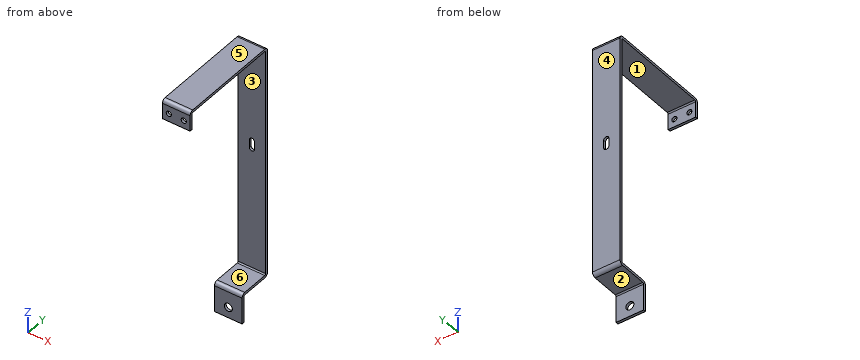
```python
from build123d import *

# Parameters (mm, degrees)
SKETCH1_W                    = 17.5
SKETCH1_H                    = 10
BASE_FLANGE1_DEPTH           = 1.6
EDGE_FLANGE1_DEPTH           = 17.5
EDGE_FLANGE2_STRIP_W         = 7.8732
EDGE_FLANGE2_STRIP_H         = 1.6
EDGE_FLANGE2_STRIP_CUT_DEPTH = 17.5
EDGE_FLANGE2_DEPTH           = 17.5
EDGE_FLANGE3_STRIP_W         = 7.8732
EDGE_FLANGE3_STRIP_H         = 1.6
EDGE_FLANGE3_STRIP_CUT_DEPTH = 17.5
EDGE_FLANGE3_DEPTH           = 17.5
F_4_CLEARANCE_HOLE1_D        = 3.2639
F_4_CLEARANCE_HOLE1_DEPTH    = 1.6
F_4_CLEARANCE_HOLE1_TIP      = 0.980574487
CUT_EXTRUDE3_DEPTH           = 1.6
EDGE_FLANGE4_STRIP_W         = 7.8732
EDGE_FLANGE4_STRIP_H         = 1.6
EDGE_FLANGE4_STRIP_CUT_DEPTH = 17.5
EDGE_FLANGE4_DEPTH           = 17.5
F_10_CLEARANCE_HOLE1_D       = 5.1054
F_10_CLEARANCE_HOLE1_DEPTH   = 7.6
F_10_CLEARANCE_HOLE1_TIP     = 1.533816902


# Sheet-metal steps are written as plain solids
with BuildPart() as part:
    # Sketch1 → Base-Flange1 (new body)
    with BuildSketch(Plane(origin=(0, 0, 0), x_dir=(1, 0, 0), z_dir=(0, 1, 0))):
        Rectangle(SKETCH1_W, SKETCH1_H)
    extrude(amount=BASE_FLANGE1_DEPTH)

    # Edge-Flange1 section (across the edge) → Edge-Flange1 (add)
    with BuildSketch(Plane(origin=(-8.75, 1.6, 5.7366), x_dir=(0, 0, -1), z_dir=(1, 0, 0))):
        with BuildLine():
            Line((-1.6, 0.7366), (-1.6, 65.4))
            Line((-1.6, 65.4), (0, 65.4))
            Line((0, 65.4), (0, 0.7366))
            ThreePointArc((0, 0.7366), (0.215745145, 0.215745145), (0.7366, 0))
            Line((0.7366, 0), (0.7366, -1.6))
            ThreePointArc((0.7366, -1.6), (-0.915625705, -0.915625705), (-1.6, 0.7366))
        make_face()
    extrude(amount=EDGE_FLANGE1_DEPTH)

    # Edge-Flange2 strip (across the edge) → Edge-Flange2 strip cut (cut)
    with BuildSketch(Plane(origin=(-8.75, 67, 5.7366), x_dir=(0, -1, 0), z_dir=(1, 0, 0))):
        with Locations((-1.6, -0.8)):
            Rectangle(EDGE_FLANGE2_STRIP_W, EDGE_FLANGE2_STRIP_H)
    extrude(amount=EDGE_FLANGE2_STRIP_CUT_DEPTH, mode=Mode.SUBTRACT)

    # Edge-Flange2 section (across the edge) → Edge-Flange2 (add)
    with BuildSketch(Plane(origin=(-8.75, 67, 5.7366), x_dir=(0, -1, 0), z_dir=(1, 0, 0))):
        with BuildLine():
            Line((0, 0.7366), (0, 147.4))
            Line((0, 147.4), (1.6, 147.4))
            Line((1.6, 147.4), (1.6, 0.7366))
            ThreePointArc((1.6, 0.7366), (1.815745145, 0.215745145), (2.3366, 0))
            Line((2.3366, 0), (2.3366, -1.6))
            ThreePointArc((2.3366, -1.6), (0.684374295, -0.915625705), (0, 0.7366))
        make_face()
    extrude(amount=EDGE_FLANGE2_DEPTH)

    # Edge-Flange3 strip (across the edge) → Edge-Flange3 strip cut (cut)
    with BuildSketch(Plane(origin=(-8.75, 65.4, -141.6634), x_dir=(0, 0, 1), z_dir=(1, 0, 0))):
        with Locations((-1.6, -0.8)):
            Rectangle(EDGE_FLANGE3_STRIP_W, EDGE_FLANGE3_STRIP_H)
    extrude(amount=EDGE_FLANGE3_STRIP_CUT_DEPTH, mode=Mode.SUBTRACT)

    # Edge-Flange3 section (across the edge) → Edge-Flange3 (add)
    with BuildSketch(Plane(origin=(-8.75, 65.4, -141.6634), x_dir=(0, 0, 1), z_dir=(1, 0, 0))):
        with BuildLine():
            Line((0, 0.7366), (0, 20.4))
            Line((0, 20.4), (1.6, 20.4))
            Line((1.6, 20.4), (1.6, 0.7366))
            ThreePointArc((1.6, 0.7366), (1.815745145, 0.215745145), (2.3366, 0))
            Line((2.3366, 0), (2.3366, -1.6))
            ThreePointArc((2.3366, -1.6), (0.684374295, -0.915625705), (0, 0.7366))
        make_face()
    extrude(amount=EDGE_FLANGE3_DEPTH)

    # #4 Clearance Hole1
    with Locations(Plane.XZ):
        with Locations((4.75, 0), (-4.75, 0)):
            Hole(F_4_CLEARANCE_HOLE1_D / 2, depth=F_4_CLEARANCE_HOLE1_DEPTH)
            with Locations((0, 0, -(F_4_CLEARANCE_HOLE1_DEPTH + F_4_CLEARANCE_HOLE1_TIP / 2))):  # 118° drill point
                Cone(0, F_4_CLEARANCE_HOLE1_D / 2, F_4_CLEARANCE_HOLE1_TIP, mode=Mode.SUBTRACT)

    # Sketch23 → Cut-Extrude3 (cut)
    with BuildSketch(Plane.XZ.offset(-65.4)):
        with BuildLine():
            Line((-1.65, -61.8268), (-1.65, -56.8268))
            ThreePointArc((-1.65, -56.8268), (0, -55.1768), (1.65, -56.8268))
            Line((1.65, -56.8268), (1.65, -61.8268))
            ThreePointArc((1.65, -61.8268), (0, -63.4768), (-1.65, -61.8268))
        make_face()
    extrude(amount=-CUT_EXTRUDE3_DEPTH, mode=Mode.SUBTRACT)

    # Edge-Flange4 strip (across the edge) → Edge-Flange4 strip cut (cut)
    with BuildSketch(Plane(origin=(8.75, 45, -141.6634), x_dir=(0, 1, 0), z_dir=(-1, 0, 0))):
        with Locations((-1.6, -0.8)):
            Rectangle(EDGE_FLANGE4_STRIP_W, EDGE_FLANGE4_STRIP_H)
    extrude(amount=EDGE_FLANGE4_STRIP_CUT_DEPTH, mode=Mode.SUBTRACT)

    # Edge-Flange4 section (across the edge) → Edge-Flange4 (add)
    with BuildSketch(Plane(origin=(8.75, 45, -141.6634), x_dir=(0, 1, 0), z_dir=(-1, 0, 0))):
        with BuildLine():
            Line((0, 0.7366), (0, 17.5))
            Line((0, 17.5), (1.6, 17.5))
            Line((1.6, 17.5), (1.6, 0.7366))
            ThreePointArc((1.6, 0.7366), (1.815745145, 0.215745145), (2.3366, 0))
            Line((2.3366, 0), (2.3366, -1.6))
            ThreePointArc((2.3366, -1.6), (0.684374295, -0.915625705), (0, 0.7366))
        make_face()
    extrude(amount=EDGE_FLANGE4_DEPTH)

    # #10 Clearance Hole1
    with Locations(Plane(origin=(0, 46.6, 0), x_dir=(1, 0, 0), z_dir=(0, 1, 0))):
        with Locations((0, 152.4)):
            Hole(F_10_CLEARANCE_HOLE1_D / 2, depth=F_10_CLEARANCE_HOLE1_DEPTH)
            with Locations((0, 0, -(F_10_CLEARANCE_HOLE1_DEPTH + F_10_CLEARANCE_HOLE1_TIP / 2))):  # 118° drill point
                Cone(0, F_10_CLEARANCE_HOLE1_D / 2, F_10_CLEARANCE_HOLE1_TIP, mode=Mode.SUBTRACT)


solid = part.part
```
Geometry check sheet. Reference: the model listing, model coordinates, mm. Face numbers are marked on the shaded views. A direction names the side the tool comes from. Round coordinates to 2 decimals unless told otherwise and drop trailing zeros. Order: outer loops, then holes, each group sorted by start corner. A loop starts at its lowest first (then second) coordinate and runs counter-clockwise, first axis right, second up. Notation, with made-up numbers: M 11.5,70 L 49.5,70 A25 ccw 49.5,87 Z; hole C 76.25,-21 d6. An arc over 180 degrees is marked long. Answer as CSV lines item,"result".
1) Gauge pin test, flat ends, axial feed: pin 1 Ø5 at (x, z) = (2, -148.5) entering from -Y; pin 2 Ø4 at (x, z) = (-4, -44.5) entering from -Y; pin 3 Ø3 at (x, z) = (0, -152.4) entering from +Y; pin 4 Ø3 at (x, y) = (-4, 57.5) entering from -Z. Record the tip position at first contact, or that the pin passes through.
Entries:
pin 1,"y = 45"
pin 2,"y = 65.4"
pin 3,"through"
pin 4,"z = -141.66"
2) Mould release check, pull along Z, two halves, no side actions. Record for the marked faces 3, 4, 5 and 6: +Z half, -Z half, draft (parallel to the pull), parting line (faces both ways), or undercut.
Entries:
face 3,"undercut"
face 4,"draft"
face 5,"+Z half"
face 6,"undercut"
3) Sectioned sample at A-A on x = 0. Record the cut outline in (y, z).
Entries:
outline,"M 0,-5 L 1.6,-5 L 1.6,5 A0.74 cw 2.34,5.74 L 64.66,5.74 A0.74 cw 65.4,5 L 65.4,-55.18 L 67,-55.18 L 67,5 A2.34 ccw 64.66,7.34 L 2.34,7.34 A2.34 ccw 0,5 Z; M 45,-159.16 L 46.6,-159.16 L 46.6,-154.95 L 45,-154.95 Z; M 45,-149.85 L 46.6,-149.85 L 46.6,-142.4 A0.74 cw 47.34,-141.66 L 64.66,-141.66 A2.34 ccw 67,-139.33 L 67,-63.48 L 65.4,-63.48 L 65.4,-139.33 A0.74 cw 64.66,-140.06 L 47.34,-140.06 A2.34 ccw 45,-142.4 Z"
4) Sectioned sample at C-C on z = 0. Record the cut outline in (x, y), and give its area (3 significant figures).
Entries:
outline,"M -8.75,0 L -6.38,0 L -6.38,1.6 L -8.75,1.6 Z; M -8.75,65.4 L 8.75,65.4 L 8.75,67 L -8.75,67 Z; M -3.12,0 L 3.12,0 L 3.12,1.6 L -3.12,1.6 Z; M 6.38,0 L 8.75,0 L 8.75,1.6 L 6.38,1.6 Z"
area,"45.6 mm2"
5) Thickness scan on probe 1 along X at (y, z) = (1, 0); probe 2 along Z at (x, y) = (-4.5, 51.5); probe 3 along Y at (x, z) = (2.75, -3). Record the ranges inside material, lowest first. Write a range as [from, to].
Entries:
probe 1,"[-8.75, -6.38], [-3.12, 3.12], [6.38, 8.75]"
probe 2,"[-141.66, -140.06], [5.74, 7.34]"
probe 3,"[0, 1.6], [65.4, 67]"
6) Sectioned sample at D-D on y = 37.5. Record the cut outline in (x, z).
Entries:
outline,"M -8.75,5.74 L 8.75,5.74 L 8.75,7.34 L -8.75,7.34 Z"
7) Tool access check on the marked faces 1 and 2. Record the directions out of +Z, -Z, +X, -X, +Y, -Y that give a thin tool (end or side, any length) a straight path to the whole face; none if there is none.
Entries:
face 1,"+X, -X"
face 2,"-Z, +X, -X, +Y"
8) Sectioned sample at B-B on z = -152.4. Record the cut outline in (x, y).
Entries:
outline,"M -8.75,45 L -2.55,45 L -2.55,46.6 L -8.75,46.6 Z; M 2.55,45 L 8.75,45 L 8.75,46.6 L 2.55,46.6 Z"
